Input: part model. Units: mm. Frame: model coordinates. Face numbers are marked on the shaded views. A direction names the side the tool comes from. Round coordinates to 2 decimals unless told otherwise and drop trailing zeros. Order: outer loops, then holes, each group sorted by start corner. A loop starts at its lowest first (then second) coordinate and runs counter-clockwise, first axis right, second up. Notation, with made-up numbers: (81.25, 78.5) -> (96.25, 78.5) arc R22 cw to (96.25, 91.5) -> close; hole circle Ø9 at (-37, 2.5). An arc over 180 degrees is marked (long way). Use a Markdown table: item, result.
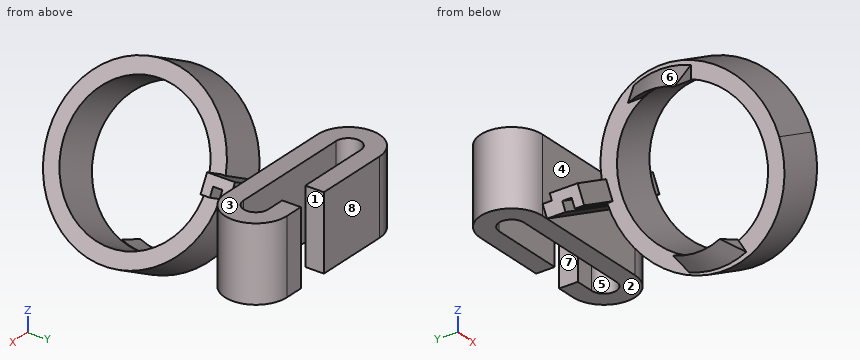
from build123d import *

# Parameters (mm, degrees)
F1_DEPTH       = 12
F5_DEPTH       = 18.5
F7_R           = 11.5
F8_DEPTH       = 8
F11_ANGLE_BACK = 20
F11_ANGLE      = 40


with BuildPart() as f1:
    # F0 (on Top) → F1 (new body)
    with BuildSketch(Plane.XY):
        with BuildLine():
            Line((0, 0), (-20, 0))
            ThreePointArc((-20, 0), (-22, 2), (-20, 4))
            Line((-20, 4), (-8, 4))
            Line((-8, 4), (-8, 7))
            Line((-8, 7), (-20, 7))
            ThreePointArc((-20, 7), (-25, 2), (-20, -3))
            Line((-20, -3), (0, -3))
            ThreePointArc((0, -3), (5, 2), (0, 7))
            Line((0, 7), (-3, 7))
            Line((-3, 7), (-3, 4))
            Line((-3, 4), (0, 4))
            ThreePointArc((0, 4), (2, 2), (0, 0))
        make_face()
    extrude(amount=F1_DEPTH)

    # F4 (on line) → F5 (join)
    with BuildSketch(Plane(origin=(-14.7844431916, 0, -7.9443702008), x_dir=(0, -1, 0), z_dir=(-0.8808807435, 0, -0.4733382677))):
        Polygon((3, 11.0186671228), (3, 9.0186671228), (6, 9.0186671228), (6, 10.5186671228), (7.5, 10.5186671228), (7.5, 9.0186671228), (9, 9.0186671228), (9, 12.0186671228), (4.5, 12.0186671228), (4.5, 11.0186671228), align=None)
    extrude(amount=-F5_DEPTH)

    # F7 (on offset) → F8 (join)
    with BuildSketch(Plane(origin=(-1.5712320387, 0, -0.8442961852), x_dir=(0, -1, 0), z_dir=(-0.8808807435, 0, -0.4733382677))):
        with BuildLine():
            ThreePointArc((36.0992396533, 9.6230288318), (24.609219733, 23.3961911411), (8.9992396533, 14.5616521217))
            Line((8.9992396533, 14.5616521217), (8.9992396533, 4.6844055418))
            ThreePointArc((8.9992396533, 4.6844055418), (24.609219733, -4.1501334776), (36.0992396533, 9.6230288318))
        make_face()
        with Locations((22.0992396533, 9.6230288318)):
            Circle(F7_R, mode=Mode.SUBTRACT)
        with BuildLine():
            Line((8.9992396533, 4.6844055418), (8.9992396533, 14.5616521217))
            ThreePointArc((8.9992396533, 14.5616521217), (8.0992396533, 9.6230288318), (8.9992396533, 4.6844055418))
        make_face()
    extrude(amount=F8_DEPTH)

    # F10 (on offset) → F11 (revolve)
    with BuildSketch(Plane.XZ.offset(21.7), mode=Mode.PRIVATE) as f11_sk:
        Polygon((-6.7922217721, -8.029286104), (-7.7298357056, -6.2843900851), (-11.4623919126, -7.7224527269), align=None)
        Polygon((-21.8758338022, 11.6569236308), (-18.6166158629, 13.9758670161), (-19.5542297964, 15.720763035), align=None)
    revolve(f11_sk.sketch.rotate(Axis((-15.3602525801, -21.7, 2.6705470646), (-0.8808807435, 0, -0.4733382677)), -F11_ANGLE_BACK), axis=Axis((-15.3602525801, -21.7, 2.6705470646), (-0.8808807435, 0, -0.4733382677)), revolution_arc=F11_ANGLE)


solid = f1.part
1) Pin query (flat end, axial travel): pin 1 Ø3.5 at (y, z) = (6, 6.5) entering from -X; pin 2 Ø1.5 at (y, z) = (6, 8.5) entering from +X; pin 3 Ø1 at (x, z) = (-14, 2) entering from -Y; pin 4 Ø3 at (x, y) = (-5, 4.5) entering from +Z. Return the tip coordinate at first contact, or that it passes through.
Results found:
| item | result |
|---|---|
| pin 1 | stops at x = -24.47 |
| pin 2 | stops at x = 3.8 |
| pin 3 | stops at y = -3 |
| pin 4 | passes through |
2) Pull-direction query (X, two-part tool) for the marked faces 6, 7 and 8; classes: +X half, -X half, draft (parallel to the pull), parting line (faces both ways), or undercut.
Results found:
| item | result |
|---|---|
| face 6 | -X half |
| face 7 | undercut |
| face 8 | draft |
3) Cut plane C-C on y = 2. Return loops of the section in (x, z), and give its area (3 significant figures).
Results found:
| item | result |
|---|---|
| outline | (-25, 0) -> (-22, 0) -> (-22, 12) -> (-25, 12) -> close; (2, 0) -> (5, 0) -> (5, 12) -> (2, 12) -> close |
| area | 72.0 mm² |
4) Line query: L1, parallel to Y at x = -17.25, z = 7.25; L2, parallel to Y at x = -15.5, z = 10.5; L3, parallel to Y at x = -8.5, z = 5. Output: solid intervals per line, ascending. Write a range as [from, to].
Results found:
| item | result |
|---|---|
| L1 | y = [-3, 0], [4, 7] |
| L2 | y = [-34.24, -31.25], [-12.95, -9.95], [-3, 0], [4, 7] |
| L3 | y = [-36.05, -33.54], [-10.66, -8.15], [-3, 0], [4, 7] |
5) Cut plane D-D on y = -6.5. Return loops of the section in (x, z).
Results found:
| item | result |
|---|---|
| outline | (-20.47, 2.64) -> (-19.76, 1.32) -> (-3.47, 10.08) -> (-4.18, 11.4) -> close |
6) Cut plane A-A on y = -14. Return loops of the section in (x, z), and give its area (3 significant figures).
Results found:
| item | result |
|---|---|
| outline | (-18.58, 13.9) -> (-17.04, 11.04) -> (-9.99, 14.82) -> (-11.53, 17.69) -> close; (-9.31, -3.35) -> (-7.77, -6.21) -> (-0.72, -2.43) -> (-2.26, 0.44) -> close |
| area | 52.1 mm² |
7) Cut plane B-B on x = -2.25. Count the separate pieces of the cut face and the enclosed holes in it, and give its area (3 significant figures).
Results found:
| item | result |
|---|---|
| separate pieces | 3 |
| enclosed holes | 0 |
| area | 135 mm² |
8) Set-up query: the marked faces 1, 2, 3, 4 and 5. Return all of +Z, -Z, +X, -X, +Y, -Y with unobstructed straight access to the full face (end or side cutting, diameter ignored); none if empty.
Results found:
| item | result |
|---|---|
| face 1 | +Z, -Z, +Y |
| face 2 | -Z, +X, -X, +Y |
| face 3 | +Z, +X, -X, +Y |
| face 4 | none |
| face 5 | +Z, -Z |
